```python
from build123d import *

# Parameters (mm, degrees)
BOSS_EXTRUDE1_DEPTH      = 5
SKETCH2_W                = 5
SKETCH2_H                = 22.5
BOSS_EXTRUDE2_DEPTH      = 38
SKETCH5_W                = 25
SKETCH5_H                = 5
BOSS_EXTRUDE3_DEPTH      = 30
FILLET3_R                = 5
SKETCH6_R                = 3
CUT_EXTRUDE4_DEPTH       = 172
SKETCH7_W                = 5
SKETCH7_H                = 22.5
BOSS_EXTRUDE4_DEPTH      = 51.5
SKETCH3_R                = 1.3
CUT_EXTRUDE2_DEPTH       = 357.71872673
SKETCH9_W                = 116
SKETCH9_H                = 63.779574991
CUT_EXTRUDE6_DEPTH       = 10
SKETCH10_W               = 25
SKETCH10_H               = 5
BOSS_EXTRUDE5_DEPTH      = 70
BOSS_EXTRUDE6_DEPTH      = 25
SKETCH12_W               = 25
SKETCH12_H               = 5
BOSS_EXTRUDE7_DEPTH      = 19.72
BOSS_EXTRUDE8_DEPTH      = 15
BOSS_EXTRUDE8_DEPTH_BACK = 4
CUT_EXTRUDE7_DEPTH       = 15
SKETCH15_R               = 2.25
CUT_EXTRUDE8_DEPTH       = 20
SKETCH16_W               = 6
SKETCH16_H               = 3
BOSS_EXTRUDE9_DEPTH      = 12.4
SKETCH17_R               = 1
CUT_EXTRUDE9_DEPTH       = 282.347152812
SKETCH27_W               = 25.232191294
SKETCH27_H               = 19
BOSS_EXTRUDE11_DEPTH     = 3
FILLET4_R                = 5
SKETCH18_R               = 2.25
CUT_EXTRUDE10_DEPTH      = 378.078044336
SKETCH19_W               = 4.5
SKETCH19_H               = 6
CUT_EXTRUDE12_DEPTH      = 383.13686347
FILLET6_R                = 10
SKETCH21_W               = 27
SKETCH21_H               = 70
CUT_EXTRUDE14_DEPTH      = 383.13686347
FILLET7_R                = 10
FILLET8_R                = 2.5
SKETCH22_R               = 2.25
CUT_EXTRUDE16_DEPTH      = 10
SKETCH23_W               = 17.043474802
SKETCH23_H               = 5.138762975
BOSS_EXTRUDE10_DEPTH     = 7
CUT_EXTRUDE17_REACH      = 372.436
CUT_EXTRUDE18_REACH      = 380.086
SKETCH25_R               = 2.25
SKETCH28_R               = 2.25
CUT_EXTRUDE19_DEPTH      = 384.936136276
CUT_EXTRUDE20_DEPTH      = 126
CUT_EXTRUDE20_DEPTH_BACK = 10
SKETCH29_W               = 186
SKETCH29_H               = 118
SKETCH30_R               = 2.25
CUT_EXTRUDE21_DEPTH      = 383.13686347


with BuildPart() as part:
    # Sketch1 → Boss-Extrude1 (new body)
    with BuildSketch(Plane(origin=(0, 0, 0), x_dir=(1, 0, 0), z_dir=(0, 1, 0))):
        Polygon((0, 0), (0, -300), (186, -300), (186, 0), (176, 0), (151, 0), (151, -56.115865257), (35, -56.115865257), (35, 0), (10, 0), align=None)
    extrude(amount=BOSS_EXTRUDE1_DEPTH)

    # Sketch2 → Boss-Extrude2 (add)
    with BuildSketch(Plane.XZ):
        with Locations((53, 82.75)):
            Rectangle(SKETCH2_W, SKETCH2_H)
        with Locations((133, 82.75)):
            Rectangle(SKETCH2_W, SKETCH2_H)
    extrude(amount=BOSS_EXTRUDE2_DEPTH)

    # Sketch5 → Boss-Extrude3 (add)
    with BuildSketch(Plane.XZ):
        with Locations((173.5, 297.5)):
            Rectangle(SKETCH5_W, SKETCH5_H)
        with Locations((173.5, 242.5)):
            Rectangle(SKETCH5_W, SKETCH5_H)
        with Locations((173.5, 187.5)):
            Rectangle(SKETCH5_W, SKETCH5_H)
        with Locations((173.5, 132.5)):
            Rectangle(SKETCH5_W, SKETCH5_H)
    extrude(amount=BOSS_EXTRUDE3_DEPTH)

    # Fillet3
    fillet3_edges = [part.edges().sort_by_distance(p)[0] for p in [
        (173.5, 0, 295),
        (173.5, 0, 240),
        (173.5, 0, 185),
        (173.5, 0, 130),
    ]]
    fillet(fillet3_edges, radius=FILLET3_R)

    # Sketch6 → Cut-Extrude4 (cut)
    with BuildSketch(Plane.XY.offset(300)):
        with Locations((178, -24)):
            Circle(SKETCH6_R)
    extrude(amount=-CUT_EXTRUDE4_DEPTH, mode=Mode.SUBTRACT)

    # Sketch7 → Boss-Extrude4 (add)
    with BuildSketch(Plane.XZ):
        with Locations((2.5, 11.25)):
            Rectangle(SKETCH7_W, SKETCH7_H)
        with Locations((183.5, 11.25)):
            Rectangle(SKETCH7_W, SKETCH7_H)
    extrude(amount=BOSS_EXTRUDE4_DEPTH)

    # Sketch3 → Cut-Extrude2 (cut, through all)
    with BuildSketch(Plane(origin=(186, 0, 0), x_dir=(0, 0, -1), z_dir=(1, 0, 0))):
        with Locations((-74, -32.9)):
            Circle(SKETCH3_R)
        with Locations((-91.5, -32.9)):
            Circle(SKETCH3_R)
        with Locations((-20, -46.4)):
            Circle(SKETCH3_R)
        with Locations((-2.5, -46.4)):
            Circle(SKETCH3_R)
    extrude(amount=-CUT_EXTRUDE2_DEPTH, mode=Mode.SUBTRACT)

    # Sketch9 → Cut-Extrude6 (cut)
    with BuildSketch(Plane.XZ):
        with Locations((93, 31.889787496)):
            Rectangle(SKETCH9_W, SKETCH9_H)
    extrude(amount=-CUT_EXTRUDE6_DEPTH, mode=Mode.SUBTRACT)

    # Sketch10 → Boss-Extrude5 (add)
    with BuildSketch(Plane.XZ.offset(30)):
        with Locations((173.5, 297.5)):
            Rectangle(SKETCH10_W, SKETCH10_H)
        with Locations((173.5, 132.5)):
            Rectangle(SKETCH10_W, SKETCH10_H)
    extrude(amount=BOSS_EXTRUDE5_DEPTH)

    # Sketch11 → Boss-Extrude6 (add)
    with BuildSketch(Plane(origin=(186, 0, 0), x_dir=(0, 0, -1), z_dir=(1, 0, 0))):
        Polygon((-300, -100), (-304.901863346, -134.643852153), (-300, -135.337431613), (-295, -100), align=None)
    extrude(amount=-BOSS_EXTRUDE6_DEPTH)

    # Sketch12 → Boss-Extrude7 (add)
    with BuildSketch(Plane.XZ.offset(100)):
        with Locations((173.5, 132.5)):
            Rectangle(SKETCH12_W, SKETCH12_H)
    extrude(amount=BOSS_EXTRUDE7_DEPTH)

    # Sketch13 → Boss-Extrude8 (add, two sides: drawn at the far end of the back side and taken through both)
    with BuildSketch(Plane(origin=(0, 0, 130), x_dir=(-1, 0, 0), z_dir=(0, 0, -1)).offset(-BOSS_EXTRUDE8_DEPTH_BACK)):
        Polygon((-186, -115.314128401), (-186, -119.72), (-161, -123.135183378), (-161, -115.314128401), align=None)
    extrude(amount=BOSS_EXTRUDE8_DEPTH + BOSS_EXTRUDE8_DEPTH_BACK)

    # Sketch14 → Cut-Extrude7 (cut)
    with BuildSketch(Plane(origin=(19.462480736, -142.470246704, 0), x_dir=(0.9907978149243063, 0.1353502491361595, 0), z_dir=(0.1353502491361595, -0.9907978149243063, 0))):
        Polygon((186.357631366, 115), (168.084261749, 132.037436989), (198.015187573, 130.430954629), (197.515117956, 111.366582762), (186.357631366, 109.607523038), align=None)
    extrude(amount=-CUT_EXTRUDE7_DEPTH, mode=Mode.SUBTRACT)

    # Sketch15 → Cut-Extrude8 (cut)
    with BuildSketch(Plane(origin=(0, 39.65203451, 280.240211564), x_dir=(1, 0, 0), z_dir=(0, 0.14009757598944012, 0.9901377021414158))):
        with Locations(Location((178, -168.031966348, 0), (0, 0, 270))):
            Circle(SKETCH15_R)
        with Locations(Location((169, -149.043043011, 0), (0, 0, 270))):
            Circle(SKETCH15_R)
    extrude(amount=-CUT_EXTRUDE8_DEPTH, mode=Mode.SUBTRACT)

    # Sketch16 → Boss-Extrude9 (add)
    with BuildSketch(Plane.XZ):
        with Locations((169, 273.5)):
            Rectangle(SKETCH16_W, SKETCH16_H)
        with Locations((140.4, 273.5)):
            Rectangle(SKETCH16_W, SKETCH16_H)
        with Locations((169, 218.5)):
            Rectangle(SKETCH16_W, SKETCH16_H)
        with Locations((169, 163.5)):
            Rectangle(SKETCH16_W, SKETCH16_H)
        with Locations((140.4, 218.5)):
            Rectangle(SKETCH16_W, SKETCH16_H)
        with Locations((140.4, 163.5)):
            Rectangle(SKETCH16_W, SKETCH16_H)
    extrude(amount=BOSS_EXTRUDE9_DEPTH)

    # Sketch17 → Cut-Extrude9 (cut, through all)
    with BuildSketch(Plane(origin=(0, 0, 162), x_dir=(-1, 0, 0), z_dir=(0, 0, -1))):
        with BuildLine():
            ThreePointArc((-169.75, -5.6), (-169.95, -6.2), (-169.75, -6.8))
            ThreePointArc((-169.75, -6.8), (-168.633772234, -7.148683298), (-167.95, -6.2))
            ThreePointArc((-167.95, -6.2), (-168.633772234, -5.251316702), (-169.75, -5.6))
        make_face()
        with Locations((-140.45, -6.2)):
            Circle(SKETCH17_R)
    extrude(amount=-CUT_EXTRUDE9_DEPTH, mode=Mode.SUBTRACT)

    # Sketch27 → Boss-Extrude11 (add)
    with BuildSketch(Plane(origin=(19.462480736, -142.470246704, 0), x_dir=(0.9907978149243063, 0.1353502491361595, 0), z_dir=(0.1353502491361595, -0.9907978149243063, 0))):
        with Locations((155.468166102, 124.5)):
            Rectangle(SKETCH27_W, SKETCH27_H)
    extrude(amount=BOSS_EXTRUDE11_DEPTH)

    # Fillet4
    fillet4_edges = [part.edges().sort_by_distance(p)[0] for p in [
        (140.4, 0, 220),
        (169, 0, 165),
        (169, 0, 220),
        (140.4, 0, 275),
        (140.4, 0, 165),
        (169, 0, 275),
    ]]
    fillet(fillet4_edges, radius=FILLET4_R)

    # Sketch18 → Cut-Extrude10 (cut, through all)
    with BuildSketch(Plane(origin=(0, -115.314128401, 0), x_dir=(1, 0, 0), z_dir=(0, 1, 0))):
        with Locations(Location((174.885718372, -120.99470656, 0), (0, 0, 180))):
            Circle(SKETCH18_R)
    extrude(amount=-CUT_EXTRUDE10_DEPTH, mode=Mode.SUBTRACT)

    # Sketch19 → Cut-Extrude12 (cut, through all)
    with BuildSketch(Plane.XZ):
        with Locations((144.95, 82.75)):
            Rectangle(SKETCH19_W, SKETCH19_H)
        with Locations((41.05, 82.75)):
            Rectangle(SKETCH19_W, SKETCH19_H)
    extrude(amount=-CUT_EXTRUDE12_DEPTH, mode=Mode.SUBTRACT)

    # Fillet6
    fillet6_edges = [part.edges().sort_by_distance(p)[0] for p in [
        (35, 2.5, 63.779574991),
        (151, 2.5, 63.779574991),
    ]]
    fillet(fillet6_edges, radius=FILLET6_R)

    # Sketch21 → Cut-Extrude14 (cut, through all)
    with BuildSketch(Plane.XZ):
        with Locations((13.5, 83)):
            Rectangle(SKETCH21_W, SKETCH21_H)
        with Locations((172.5, 83)):
            Rectangle(SKETCH21_W, SKETCH21_H)
    extrude(amount=-CUT_EXTRUDE14_DEPTH, mode=Mode.SUBTRACT)

    # Fillet7
    fillet7_edges = [part.edges().sort_by_distance(p)[0] for p in [
        (27, 2.5, 118),
        (27, 2.5, 48),
        (159, 2.5, 48),
        (159, 2.5, 118),
    ]]
    fillet(fillet7_edges, radius=FILLET7_R)

    # Fillet8
    fillet8_edges = [part.edges().sort_by_distance(p)[0] for p in [
        (55.5, 0, 82.75),
        (130.5, 0, 82.75),
    ]]
    fillet(fillet8_edges, radius=FILLET8_R)

    # Sketch22 → Cut-Extrude16 (cut)
    with BuildSketch(Plane.XZ):
        with Locations(Location((123, 76.044790491, 0), (0, 0, 270))):
            Circle(SKETCH22_R)
        with Locations(Location((63, 76.044790491, 0), (0, 0, 270))):
            Circle(SKETCH22_R)
        with Locations(Location((24.5, 25.25, 0), (0, 0, 270))):
            Circle(SKETCH22_R)
        with Locations(Location((161.5, 25.617459027, 0), (0, 0, 270))):
            Circle(SKETCH22_R)
    extrude(amount=-CUT_EXTRUDE16_DEPTH, mode=Mode.SUBTRACT)

    # Sketch23 → Boss-Extrude10 (add)
    with BuildSketch(Plane.XY.offset(135)):
        with Locations((169.584553608, -121.006176699)):
            Rectangle(SKETCH23_W, SKETCH23_H)
    extrude(amount=BOSS_EXTRUDE10_DEPTH)

    # Sketch24 → Cut-Extrude17 (cut, up to next)
    with BuildSketch(Plane.ZY.offset(-161.062816207), mode=Mode.PRIVATE) as cut_extrude17_sk1:
        Polygon((142, -121.648432415), (135, -122.638883571), (134.714975443, -124.33810847), (142, -124.33810847), align=None)
    cut_extrude17_tool1 = extrude(cut_extrude17_sk1.sketch, amount=-CUT_EXTRUDE17_REACH, mode=Mode.PRIVATE) & part.part
    add(cut_extrude17_tool1.solids().sort_by_distance((161.062816, -123.230784, 138.703404))[0], mode=Mode.SUBTRACT)

    # Cut-Extrude18: up to this plane
    cut_extrude18_end = Plane(origin=(186.407050747, -121.648432415, 142), z_dir=(0, 0.9901377021414159, -0.1400975759894394))
    # Sketch25 → Cut-Extrude18 (cut, up to the surface)
    with BuildSketch(Plane(origin=(0, -118.436795211, 0), x_dir=(1, 0, 0), z_dir=(0, 1, 0)), mode=Mode.PRIVATE) as cut_extrude18_sk1:
        with Locations(Location((174.719138996, -138.089405518, 0), (0, 0, 270))):
            Circle(SKETCH25_R)
    cut_extrude18_tool1 = split(extrude(cut_extrude18_sk1.sketch, amount=-CUT_EXTRUDE18_REACH, mode=Mode.PRIVATE), bisect_by=cut_extrude18_end, keep=Keep.BOTH, mode=Mode.PRIVATE)
    add(cut_extrude18_tool1.solids().sort_by_distance((174.719139, -118.436795, 138.089406))[0], mode=Mode.SUBTRACT)

    # Sketch28 → Cut-Extrude19 (cut, through all)
    with BuildSketch(Plane(origin=(0, 5, 0), x_dir=(1, 0, 0), z_dir=(0, 1, 0))):
        with Locations(Location((93, -260, 0), (0, 0, 270))):
            Circle(SKETCH28_R)
    extrude(amount=-CUT_EXTRUDE19_DEPTH, mode=Mode.SUBTRACT)

    # Sketch29 → Cut-Extrude20 (cut, two sides: drawn at the far end of the back side and taken through both)
    with BuildSketch(Plane.XZ.offset(-CUT_EXTRUDE20_DEPTH_BACK)):
        with Locations((93, 59)):
            Rectangle(SKETCH29_W, SKETCH29_H)
    extrude(amount=CUT_EXTRUDE20_DEPTH + CUT_EXTRUDE20_DEPTH_BACK, mode=Mode.SUBTRACT)

    # Sketch30 → Cut-Extrude21 (cut, through all)
    with BuildSketch(Plane.XZ):
        with Locations(Location((65, 138, 0), (0, 0, 270))):
            Circle(SKETCH30_R)
        with Locations(Location((121, 138, 0), (0, 0, 270))):
            Circle(SKETCH30_R)
    extrude(amount=-CUT_EXTRUDE21_DEPTH, mode=Mode.SUBTRACT)


solid = part.part
```
The listing builds one solid part. Answer for the finished solid, in the listing's coordinates (mm). A direction names the side the tool comes from. Coordinates: 2 decimals unless noted, no trailing zeros. Order: outer loops, then holes, each group sorted by start corner. A loop starts at its lowest first (then second) coordinate and runs counter-clockwise, first axis right, second up. Notation, with made-up numbers: M 31,36 L 70,36 A17 cw 70,57 Z; hole C 38,6 d9. An arc over 180 degrees is marked long. Answer as a JSON object with one key per item and string values. Group by question number.
1. Flat-ended cylindrical pins translate along their axes: P1, Ø4, axis at y = -4.5, z = 165, coming from the +X side; P2, Ø1.5, axis at x = 89.5, z = 215, coming from the -Y side; P3, Ø1.5, axis at x = 171, y = -122, coming from the -Z side. Find the tip coordinate at first contact, or state that the pin passes through.
2. Section A-A on y = -24 is taken. State how many separate pieces and enclosed holes the cut face has, then the cut area to 3 significant figures.
3. Section B-B on x = 38.5 is taken. Write down the section's boundary in (y, z).
4. Section D-D on z = 209.5 is taken. Write down the section's boundary in (x, y), then the cut area to 3 significant figures.
5. A tool of negligible diameter and unlimited length cuts with its end or side. For faces 5 (the cylindrical face through (175.8, -126.6, 301.3)), 6 (the flat face through (140, -9, 220)), 7 (the flat face through (173, -115.314, 124)), 8 (the flat face through (172, -5, 218)), from which of +Z, -Z, +X, -X, +Y, -Y can it reach the whole face along a straight path? Write none if from no direction.
6. Section C-C on z = 237.5 is taken. Write down the section's boundary in (x, y).
7. Determine the mould class of faces 1 (the cylindrical face through (140, -1, 277)), 2 (the flat face through (172, -5, 273)), 3 (the flat face through (92, 2, 118)), 4 (the cylindrical face through (174, -2, 239)) for opening direction Z: released by +Z, released by -Z, zero draft, split by the parting line, or undercut.
8. Straight lines are drawn through the part: line 1 (Y direction, x = 178, z = 187.4); line 2 (X direction, y = 3.9, z = 138); line 3 (X direction, y = -6, z = 218). For each, find the intervals that lie inside material, in ascending order.
Values follow:
{
 "1": {"P1": "x = 172", "P2": "y = 0", "P3": "z = 118"},
 "2": {"separate pieces": "8", "enclosed holes": "0", "area": "380 mm2"},
 "3": {"outline": "M 0,118 L 5,118 L 5,300 L 0,300 Z"},
 "4": {"outline": "M 0,0 L 186,0 L 186,5 L 0,5 Z", "area": "930 mm2"},
 "5": {"face 5": "none", "face 6": "+X, -X, -Y", "face 7": "-Z, +X, -X", "face 8": "+X, -Y"},
 "6": {"outline": "M 0,0 L 161,0 L 161,-0.67 L 186,-0.67 L 186,5 L 0,5 Z"},
 "7": {"face 1": "released by +Z", "face 2": "undercut", "face 3": "released by -Z", "face 4": "undercut"},
 "8": {"line 1": "-30 to -27, -21 to 5", "line 2": "0 to 62.75, 67.25 to 118.75, 123.25 to 186", "line 3": "137.4 to 139.47, 141.43 to 143.4, 166 to 167.97, 169.93 to 172"}
}
